Could you check a few things on this model? Use its own coordinates, in mm. A direction names the side the tool comes from. Give positions to 0.01 mm unless a question says otherwise; leave off trailing zeros. Loops run counter-clockwise (first coordinate to the right, second up) from the corner with the lowest first, then second, coordinate; pieces in that order, holes last. Notation, with made-up numbers: (-16.5, -38.5) - (42.5, -38.5) arc R15 cw to (42.5, -30.5) - close; hole circle Ø6 at (32.5, 74). An arc over 180 degrees is marked (long way). Write each question's results on one line, items separated by ' | '. Start each with the question number.
Autodesk Inventor part; units mm, degrees
ref_plane "YZ Plane" through (0, 0, 0) normal (1, 0, 0) x (0, 1, 0)
ref_plane "XZ Plane" through (0, 0, 0) normal (0, 1, 0) x (-1, 0, 0)
ref_plane "XY Plane" through (0, 0, 0) normal (0, 0, 1) x (1, 0, 0)
sketch "Sketch14" plane through (0, 0, 0) normal (0, 0, 1) x (1, 0, 0)
  line L0 (-139.2442, -85) -> (-139.2442, -47.3019)
  line L1 (0, 0) -> (0, -356.2475) construction
  line L2 (0, 0) -> (-146.5249, 0) construction
  circle A0 centre (0, -228.6) radius 228.6 construction
  arc A1 (0, 0) -> (-139.2442, -47.3019) centre (0.2992, -229.4806) ccw
  arc A2 (0, -28.6152) -> (-139.2442, -85) centre (0.2992, -229.4806) ccw
  line L3 (139.2442, -85) -> (139.2442, -47.3019)
  arc A3 (139.2442, -47.3019) -> (0, 0) centre (-0.2992, -229.4806) ccw
  arc A4 (139.2442, -85) -> (0, -28.6152) centre (-0.2992, -229.4806) ccw
  circle A5 centre (0, -15) radius 7.5
  circle A6 centre (-124, -55) radius 7.5
  circle A7 centre (124, -55) radius 7.5
  circle A8 centre (-124, -55) radius 2.5
  circle A9 centre (0, -15) radius 2.5
  circle A10 centre (124, -55) radius 2.5
  dimension "d152" = 139.2442
  dimension "d153" = 85
  dimension "d155" = 457.2
  dimension "d156" = 200.8656
  dimension "d159" = 15
  dimension "d160" = 15
  dimension "d161" = 15
  dimension "d162" = 55
  dimension "d163" = 124
  dimension "d164" = 5
  dimension "d165" = 5
  dimension "d166" = 5
extrude "Extrusion14" add sketch "Sketch14" along normal blind 5 contours L0 A1 A3 L3 A4 A2 | A5 | A6 | A7
fillet "Fillet2" radius 2 3 edges at (-126.5, -55, 5) (-2.5, -15, 5) (121.5, -55, 5)
properties part number "BaseCover" material "ABS Plastic"
Q1. I want a section at C-C, the plane z = 1.25. List the corners of the cut face in (x, y) for me, then the cut area to 3 significant figures.
Q2. I want a section at D-D, the plane y = -34. List the corners of the cut face in (x, z) for me.
Q3. If we mould it in two halves opening along X, with no side actions, what happens to faces 1 (the face through (-76.09, -43.707, 2.465)), 2 (the face through (-1, -23, 0)), 3 (the face through (72.52, -11.86, 2.46))? For each: +X half, -X half, draft (parallel to the pull), parting line (faces both ways), or undercut.
Q4. Which directions (+Z, -Z, +X, -X, +Y, -Y) give clear straight access to the entire face, cutting with the end or side of a thin tool? Please do faces 4 (the face through (74.1, -42.9, 2.5)), 5 (the face through (-0.54, -12.56, 1.48)).
Q5. I want a section at A-A, the plane y = -15. List the corners of the cut face in (x, z) for me, then the cut area to 3 significant figures.
Q6. I'm going to push flat-ended pins straight in: pin 1 Ø3 at (x, z) = (-82.5, 3) entering from +Y; pin 2 Ø1.5 at (x, z) = (-7, 2.5) entering from +Y; pin 3 Ø8 at (x, y) = (124, -55) entering from +Z. Where does each tip first touch, or does it pass through?
Q7. I need wall thicknesses on L1, parallel to Y at x = 0, z = 1.5; L2, parallel to X at y = -48, z = 3.95; L3, parallel to X at y = -69.5, z = 1.7. Which ranges of each line are inside material? Lowest first, please. Write a range as from..to.
Q8. I want a section at B-B, the plane x = -124. List the corners of the cut face in (y, z) for me.
Conclusion:
1) outline: (-139.24, -85) arc R200.87 cw to (0, -28.62) arc R200.87 cw to (139.24, -85) - (139.24, -47.3) arc R229.48 ccw to (0, 0) arc R229.48 ccw to (-139.24, -47.3) - close; hole circle Ø5 at (-124, -55); hole circle Ø5 at (0, -15); hole circle Ø5 at (124, -55) | area: 8,620 mm^2
2) outline: (-119.9, 0) - (-45.9, 0) - (-45.9, 5) - (-119.9, 5) - close; (45.9, 0) - (119.9, 0) - (119.9, 5) - (45.9, 5) - close
3) face 1: undercut | face 2: draft | face 3: +X half
4) face 4: +Z, -Z, -Y | face 5: +Z, -Z
5) outline: (-81.31, 0) - (-2.5, 0) - (-2.5, 3) arc R2 ccw to (-4.5, 5) - (-81.31, 5) - close; (2.5, 0) - (81.31, 0) - (81.31, 5) - (4.5, 5) arc R2 ccw to (2.5, 3) - close | area: 786 mm^2
6) pin 1: y = -14.88 | pin 2: y = -0.09 | pin 3: z = 4.94
7) L1: -28.62..-17.5, -12.5..0 | L2: -139.24..-85.79, 85.79..139.24 | L3: -139.24..-121.16, 121.16..139.24
8) outline: (-71.69, 0) - (-57.5, 0) - (-57.5, 3) arc R2 ccw to (-59.5, 5) - (-71.69, 5) - close; (-52.5, 0) - (-36.58, 0) - (-36.58, 5) - (-50.5, 5) arc R2 ccw to (-52.5, 3) - close
